Input: dimensioned drawing with shaded views. Units: mm. Origin: part minimum x, y, z. A direction names the side the tool comes from. Round coordinates to 2 decimals unless told otherwise and drop trailing zeros. Loops run counter-clockwise (first coordinate to the right, second up) from the corner with the lowest first, then second, coordinate; pieces in that order, holes last. Notation, with made-up numbers: M -33,42 L -13,42 A34 ccw -13,72 Z; hole C 13.25,-33 d10. An arc over 180 degrees is marked long. Answer as a JSON object with one key per item and string values.
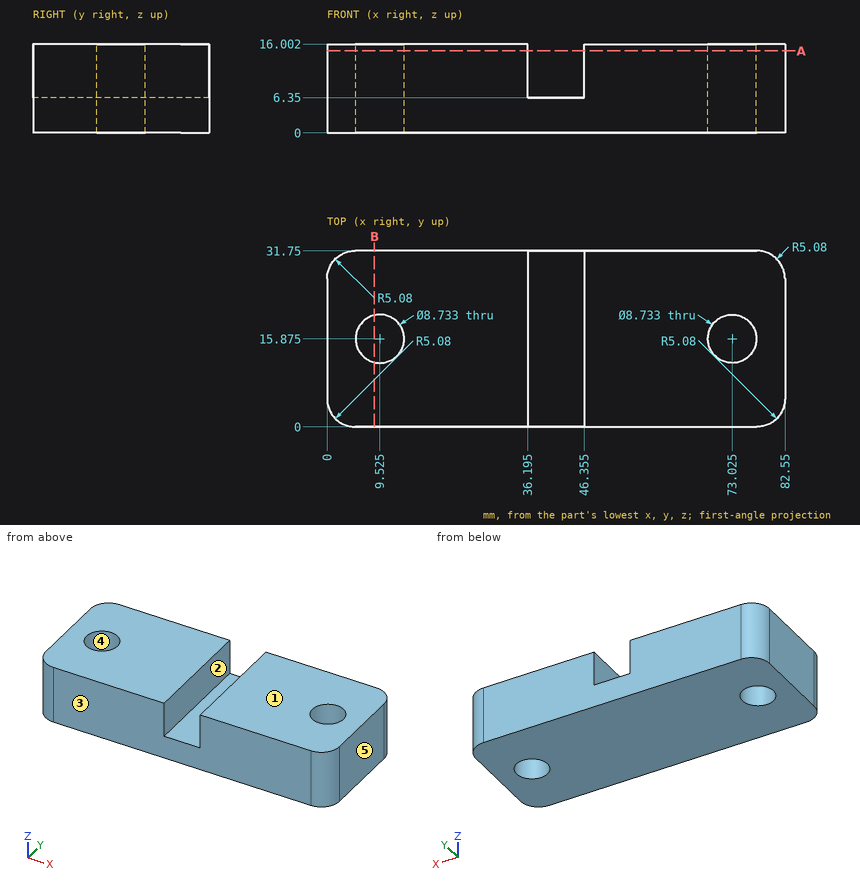
Item 1: Section B-B on x = 8.5. Return the cut outline in (y, z), then the cut area to 3 significant figures.
Answer sheet:
{"outline": "M 0,0 L 11.63,0 L 11.63,16 L 0,16 Z; M 20.12,0 L 31.75,0 L 31.75,16 L 20.12,16 Z", "area": "372 mm²"}
Item 2: Access query for the marked faces 1 and 2. Directions: +Z, -Z, +X, -X, +Y, -Y. A direction counts if a zero-diameter tool reaches every point of the face in a straight line with its end or side. Return the directions, or none.
Answer sheet:
{"face 1": "+Z, +X, -X, +Y, -Y", "face 2": "+Z, +Y, -Y"}
Item 3: Section A-A on z = 14.75. Give the number of separate pieces and of enclosed holes in the cut face, then the cut area to 3 significant figures.
Answer sheet:
{"separate pieces": "2", "enclosed holes": "2", "area": "2,160 mm²"}
Item 4: Contact query for flat-ended pins moving along their axis: pin 1 Ø5 at (x, y) = (73.025, 15.875) entering from +Z; pin 2 Ø8 at (x, y) = (40.5, 18) entering from +Z. Output: stop coordinate, or through.
Answer sheet:
{"pin 1": "passes through", "pin 2": "stops at z = 6.35"}
Item 5: Line query: probe 1 along Z at (x, y) = (43, 9); probe 2 along Y at (x, z) = (5, 11.75); probe 3 along X at (y, z) = (27.5, 8.75) (1 decimal). Output: solid intervals per line, ascending. Write a range as from..to.
Answer sheet:
{"probe 1": "z = 0..6.35", "probe 2": "y = 0..31.75", "probe 3": "x = 0.1..36.2, 46.4..82.5"}
Item 6: Pull-direction query (X, two-part tool) for the marked faces 3, 4 and 5; classes: pulls with the +X half, pulls with the -X half, needs draft (parallel to the pull), parting line crosses it, or undercut.
Answer sheet:
{"face 3": "needs draft", "face 4": "undercut", "face 5": "pulls with the +X half"}
